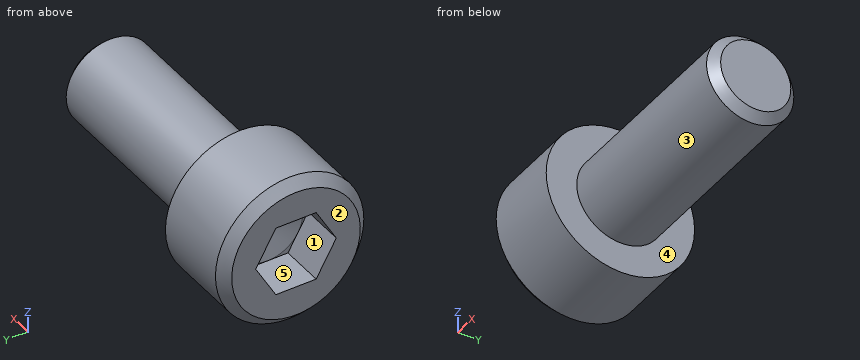
from build123d import *

# Parameters (mm, degrees)
CUT_EXTRUDE_1_DEPTH = 2.5


with BuildPart() as part:
    # 草圖1 → 旋轉1 (revolve)
    with BuildSketch(Plane.XY, mode=Mode.PRIVATE) as revolve_1_sk:
        Polygon((-5, 0), (-5, 3.683333333), (-4.433333333, 4.25), (0, 4.25), (0, 2.5), (11.5095, 2.5), (12, 2.0095), (12, 0), align=None)
    revolve(revolve_1_sk.sketch.rotate(Axis((12, 0, 0), (-1, 0, 0)), 270), axis=Axis((12, 0, 0), (-1, 0, 0)))

    # 草圖2 → 除料-旋轉1 (revolve, cut)
    with BuildSketch(Plane.XY, mode=Mode.PRIVATE) as cut_revolve_1_sk:
        Polygon((-5, 0), (-5, 2), (-2.5, 2), (-1.964101615, 0), align=None)
    revolve(cut_revolve_1_sk.sketch.rotate(Axis((-1.964101615, 0, 0), (-1, 0, 0)), 270), axis=Axis((-1.964101615, 0, 0), (-1, 0, 0)), mode=Mode.SUBTRACT)

    # 草圖3 → 除料-伸長1 (cut)
    with BuildSketch(Plane(origin=(-5, 0, 0), x_dir=(0, 0, -1), z_dir=(1, 0, 0))):
        Polygon((-2, 1.154700538), (-2, -1.154700538), (0, -2.309401077), (2, -1.154700538), (2, 1.154700538), (0, 2.309401077), align=None)
    extrude(amount=CUT_EXTRUDE_1_DEPTH, mode=Mode.SUBTRACT)


solid = part.part
Geometry check sheet. Reference: the model listing, model coordinates, mm. Face numbers are marked on the shaded views. A direction names the side the tool comes from. Coordinates: 2 decimals unless noted, no trailing zeros. Order: outer loops, then holes, each group sorted by start corner. A loop starts at its lowest first (then second) coordinate and runs counter-clockwise, first axis right, second up. Notation, with made-up numbers: (35.25, 55) - (90.25, 55) arc R12 cw to (90.25, 63) - close; hole circle Ø10 at (-39, -34). An arc over 180 degrees is marked (long way). Answer in a Markdown table with one row per item. Add a question column.
1) Gauge pin test, flat ends, axial feed: P1, Ø1, axis at x = 10, z = 1, coming from the -Y side; P2, Ø1, axis at x = 9, y = 1, coming from the -Z side; P3, Ø5, axis at x = 2, y = 2.5, coming from the +Z side. Record the tip position at first contact, or that the pin passes through.
2) Release check for a two-part mould opening along Z. For the marked faces 3, 4 and 5 record: +Z half, -Z half, draft (parallel to the pull), parting line (faces both ways), or undercut.
3) Cross-section at A-A, the plane x = 9. Record the cut outline in (y, z).
4) Set-up check for the marked faces 1 and 2: record each of +Z, -Z, +X, -X, +Y, -Y from which the full face is reachable in a straight line by a thin tool's end or side.
5) Cross-section at B-B, the plane x = -1.25. Record the cut outline in (y, z), then the cut area to 3 significant figures.
6) Material ranges on line 1 along X through (y, z) = (3, 1.25); line 2 along Y through (x, z) = (6.5, -1.5); line 3 along X through (y, z) = (0.5, 1.5), recorded low to high. Write a range as [from, to].
Check result:
| question | item | result |
|---|---|---|
| 1 | P1 | stops at y = -2.45 |
| 1 | P2 | stops at z = -2.45 |
| 1 | P3 | stops at z = 4.13 |
| 2 | face 3 | parting line |
| 2 | face 4 | draft |
| 2 | face 5 | undercut |
| 3 | outline | circle Ø5 at (0, 0) |
| 4 | face 1 | -X |
| 4 | face 2 | +Z, -Z, -X, +Y, -Y |
| 5 | outline | circle Ø8.5 at (0, 0) |
| 5 | area | 56.7 mm² |
| 6 | line 1 | x = [-5, 0] |
| 6 | line 2 | y = [-2, 2] |
| 6 | line 3 | x = [-2.39, 12] |
